Autodesk Fusion 360 part; units mm, degrees
sketch "Base Bell Crank" plane through (0, 0, 0) normal (0, 1, 0) x (1, 0, 0)
  circle A0 centre (64.9712, 0) radius 3.175
  circle A1 centre (-86.6283, 0) radius 3.175
  circle A2 centre (0, -63.5) radius 2.3813
  circle A3 centre (0, 0) radius 3.175
  line L0 (0, -63.5) -> (0, 0) construction
  line L1 (0, 0) -> (64.9712, 0) construction
  line L2 (0, 0) -> (-86.6283, 0) construction
  line L3 (-12.7, -76.2) -> (12.7, -76.2)
  line L4 (12.7, -76.2) -> (84.0212, -12.7)
  line L5 (-105.6783, 12.7) -> (-105.6783, -12.7)
  line L6 (0, -63.5) -> (0, -76.2) construction
  line L7 (64.9712, 0) -> (84.0212, 0) construction
  line L8 (84.0212, -12.7) -> (84.0212, 12.7)
  line L9 (-105.6783, 12.7) -> (84.0212, 12.7)
  line L10 (-105.6783, -12.7) -> (-12.7, -76.2)
  dimension "d12" = 4.7625
  dimension "d13" = 6.35
  dimension "d19" = 6.35
  dimension "d20" = 63.5
  dimension "d21" = 64.9712
  dimension "d22" = 86.6283
  dimension "d48" = 25.4
  dimension "d54" = 12.7
  dimension "d56" = 12.7
  dimension "d58" = 12.7
  dimension "d87" = 19.05
  dimension "d88" = 19.05
sketch "Sketch3" plane through (0, 0, 0) normal (0, 1, 0) x (1, 0, 0)
  line L0 (12.7, -76.2) -> (84.0212, -12.7)
  line L1 (0, -63.5) -> (0, 0)
  line L2 (0, 0) -> (64.9712, 0)
  line L3 (9.525, -53.5204) -> (9.525, -12.7)
  line L4 (9.525, -12.7) -> (55.3732, -12.7)
  line L5 (55.3732, -12.7) -> (9.525, -53.5204)
  line L6 (-9.525, -12.7) -> (-71.9004, -12.7)
  line L7 (-71.9004, -12.7) -> (-9.525, -55.2996)
  line L8 (-9.525, -55.2996) -> (-9.525, -12.7)
  line L9 (-105.6783, -12.7) -> (-12.7, -76.2)
  line L10 (-105.6783, 12.7) -> (84.0212, 12.7)
  line L11 (-9.525, -55.2996) -> (9.525, -53.5204) construction
  point P0 (0, -54.41)
  dimension "d93" = 19.05
  dimension "d96" = 19.05
  dimension "d98" = 25.4
  dimension "d103" = 19.05
  dimension "d104" = 25.4
extrude "Extrude1" add sketch "Base Bell Crank" along normal blind 3.175
extrude "Extrude2" cut sketch "Sketch3" along normal up to surface (3.175 mm away)
fillet "Fillet1" radius 2.54 6 edges at (-71.9004, 1.5875, 12.7) (-9.525, 1.5875, 12.7) (-9.525, 1.5875, 55.2996) (9.525, 1.5875, 53.5204) (9.525, 1.5875, 12.7) (55.3732, 1.5875, 12.7)
fillet "Fillet2" radius 6.35 2 edges at (12.7, 1.5875, 76.2) (84.0212, 1.5875, 12.7)
fillet "Fillet2" radius 6.35 2 edges at (-105.6783, 1.5875, -12.7) (84.0212, 1.5875, -12.7)
fillet "Fillet2" radius 6.35 2 edges at (-12.7, 1.5875, 76.2) (-105.6783, 1.5875, 12.7)
equation "AngleUp = 20 deg"
equation "AngleDown = 15 deg"
equation "EyeBoltRadius = 1.4 in"
equation "EBDistCC = ( AngleUp * 3.1415 * 2 * EyeBoltRadius ) / 360 deg"
equation "EBDistCCW = ( AngleDown * 3.1415 * 2 * EyeBoltRadius ) / 360 deg"
equation "TopHoletoPivot = 2.5 in"
equation "BellCrankAngleDown = ( EBDistCCW * 360 deg ) / ( TopHoletoPivot * 3.1415 * 2 )"
equation "BellCrankAngleUp = ( EBDistCC * 360 deg ) / ( TopHoletoPivot * 3.1415 * 2 )"
equation "PullDist = 0.5 in"
equation "RightHoleDist = ( PullDist * 360 deg ) / ( 3.1415 * 2 * BellCrankAngleUp )"
equation "LeftHoleDist = ( PullDist * 360 deg ) / ( 3.1415 * 2 * BellCrankAngleDown )"
equation "d12 = TopHoleOD"
equation "d13 = CableHoleOD"
equation "TopHoleOD = ( 3 / 16 ) * 1 in"
equation "CableHoleOD = 0.25 in"
equation "StrutHoleOD = 0.25 in"
equation "d19 = StrutHoleOD"
equation "d20 = TopHoletoPivot"
equation "d21 = RightHoleDist"
equation "d22 = LeftHoleDist"
equation "d37 = ( 3 / 8 ) * 1 in"
equation "d39 = ( 3 / 8 ) * 1 in"
equation "d41 = ( 3 / 8 ) * 1 in"
equation "d83 = ( 3 / 8 ) * 1 in"
CAD build for the part. Positions are in the model's coordinates, mm. A direction names the side the tool comes from. Round coordinates to 2 decimals unless told otherwise and drop trailing zeros. Order: outer loops, then holes, each group sorted by start corner. A loop starts at its lowest first (then second) coordinate and runs counter-clockwise, first axis right, second up.
Q1. Slice it at D-D (x = -56.5). Write the cut outline in (y, z) (3 decimals), and give its area (3 significant figures).
Q2. Drop a flat-ended pin along its axis: pin 1 (1 mm diameter, centred on x = -45.5, y = 1, fed in from +Z). Give the stop position or say it passes through.
Q3. Two-plate mould, pull along Z, no slides. Class faces 1 (the flat face through (-12, 0, 11)), 2 (the cylindrical face through (-104.964, 1.61, 12.274)), 3 (the flat face through (-39.665, 1.565, 34.715)): pulls with the +Z half, pulls with the -Z half, needs draft (parallel to the pull), parting line crosses it, or undercut.
Q4. Slice it at C-C (z = 24). Write the cut outline in (x, y) (3 decimals), and give its area (3 significant figures).
Q5. Which spindle directions (+Z, -Z, +X, -X, +Y, -Y) get a long thin tool onto all of the face, cutting with end or side? Do faces 4 (the flat face through (-12, 3.175, 11)), 5 (the flat face through (32.328, 1.565, 33.218)). Say none if no direction does.
Q6. Slice it at B-B (y = 1.2). State how many separate pieces and enclosed holes the cut face has, and give its area (3 significant figures).
Q7. Slice it at A-A (x = 0). Write the cut outline in (y, z) (3 decimals).
Q8. Wall check: L1, parallel to X at y = 2.25, z = 0 (3 decimals); L2, parallel to Z at x = 0, y = 1.4 (3 decimals); L3, parallel to Z at x = 1.5, y = 2.4. Give the ranges that are in metal, low to high.
Results below:
1. outline: (0, -12.7) - (3.175, -12.7) - (3.175, 12.7) - (0, 12.7) - close; (0, 23.218) - (3.175, 23.218) - (3.175, 46.287) - (0, 46.287) - close
1. area: 154 mm2
2. pin 1: stops at z = 54.14
3. face 1: needs draft
3. face 2: pulls with the +Z half
3. face 3: undercut
4. outline: (-89.133, 0) - (-55.355, 0) - (-55.355, 3.175) - (-89.133, 3.175) - close; (-9.525, 0) - (9.525, 0) - (9.525, 3.175) - (-9.525, 3.175) - close; (42.681, 0) - (71.329, 0) - (71.329, 3.175) - (42.681, 3.175) - close
4. area: 259 mm2
5. face 4: +Z, -Z, +X, -X, +Y
5. face 5: +Y, -Y
6. separate pieces: 1
6. enclosed holes: 6
6. area: 9,290 mm2
7. outline: (0, -12.7) - (3.175, -12.7) - (3.175, -3.175) - (0, -3.175) - close; (0, 3.175) - (3.175, 3.175) - (3.175, 61.119) - (0, 61.119) - close; (0, 65.881) - (3.175, 65.881) - (3.175, 76.2) - (0, 76.2) - close
8. L1: x = -105.678 to -89.803, -83.453 to -3.175, 3.175 to 61.796, 68.146 to 84.021
8. L2: z = -12.7 to -3.175, 3.175 to 61.119, 65.881 to 76.2
8. L3: z = -12.7 to -2.8, 2.8 to 61.65, 65.35 to 76.2
